from build123d import *

# Parameters (mm, degrees)
SKETCH3_R           = 7.5
SKETCH3_R_2         = 2.75
SKETCH3_W           = 30
SKETCH3_H           = 5.4
BOSS_EXTRUDE1_DEPTH = 5.4


with BuildPart() as part:
    # Sketch3 → Boss-Extrude1 (new body)
    with BuildSketch(Plane.XY):
        with BuildLine():
            Line((-242.5, 50), (207.5, 50))
            ThreePointArc((207.5, 50), (257.5, 0), (207.5, -50))
            Line((207.5, -50), (-242.5, -50))
            ThreePointArc((-242.5, -50), (-292.5, 0), (-242.5, 50))
        make_face()
        with Locations((-242.5, 0)):
            Circle(SKETCH3_R, mode=Mode.SUBTRACT)
        with Locations((207.5, 0)):
            Circle(SKETCH3_R, mode=Mode.SUBTRACT)
        with Locations((-226.332108181, 6.696960066)):
            Circle(SKETCH3_R_2, mode=Mode.SUBTRACT)
        with Locations((-226.332108181, -6.696960066)):
            Circle(SKETCH3_R_2, mode=Mode.SUBTRACT)
        with Locations((-235.803039934, -16.167891819)):
            Circle(SKETCH3_R_2, mode=Mode.SUBTRACT)
        with Locations((-249.196960066, -16.167891819)):
            Circle(SKETCH3_R_2, mode=Mode.SUBTRACT)
        with Locations((-258.667891819, -6.696960066)):
            Circle(SKETCH3_R_2, mode=Mode.SUBTRACT)
        with Locations((-258.667891819, 6.696960066)):
            Circle(SKETCH3_R_2, mode=Mode.SUBTRACT)
        with Locations((-249.196960066, 16.167891819)):
            Circle(SKETCH3_R_2, mode=Mode.SUBTRACT)
        with Locations((-235.803039934, 16.167891819)):
            Circle(SKETCH3_R_2, mode=Mode.SUBTRACT)
        with Locations((-134.5, -24)):
            Circle(SKETCH3_R_2, mode=Mode.SUBTRACT)
        with Locations((-154.5, -24)):
            Circle(SKETCH3_R_2, mode=Mode.SUBTRACT)
        with Locations((-168.5, -10)):
            Circle(SKETCH3_R_2, mode=Mode.SUBTRACT)
        with Locations((-168.5, 10)):
            Circle(SKETCH3_R_2, mode=Mode.SUBTRACT)
        with Locations((-154.5, 24)):
            Circle(SKETCH3_R_2, mode=Mode.SUBTRACT)
        with Locations((-134.5, 24)):
            Circle(SKETCH3_R_2, mode=Mode.SUBTRACT)
        with Locations((199.5, -24)):
            Circle(SKETCH3_R_2, mode=Mode.SUBTRACT)
        with Locations((219.5, -24)):
            Circle(SKETCH3_R_2, mode=Mode.SUBTRACT)
        with Locations((233.5, -10)):
            Circle(SKETCH3_R_2, mode=Mode.SUBTRACT)
        with Locations((233.5, 10)):
            Circle(SKETCH3_R_2, mode=Mode.SUBTRACT)
        with Locations((219.5, 24)):
            Circle(SKETCH3_R_2, mode=Mode.SUBTRACT)
        with Locations((199.5, 24)):
            Circle(SKETCH3_R_2, mode=Mode.SUBTRACT)
        with BuildLine():
            Line((115, 15), (150, 15))
            ThreePointArc((150, 15), (165, 0), (150, -15))
            Line((150, -15), (115, -15))
            ThreePointArc((115, -15), (100, 0), (115, 15))
        make_face(mode=Mode.SUBTRACT)
        with Locations((-227.5, 42.3)):
            Rectangle(SKETCH3_W, SKETCH3_H, mode=Mode.SUBTRACT)
        with Locations((-167.5, 42.3)):
            Rectangle(SKETCH3_W, SKETCH3_H, mode=Mode.SUBTRACT)
        with BuildLine():
            Line((14.924, 15), (49.924, 15))
            ThreePointArc((49.924, 15), (64.924, 0), (49.924, -15))
            Line((49.924, -15), (14.924, -15))
            ThreePointArc((14.924, -15), (-0.076, 0), (14.924, 15))
        make_face(mode=Mode.SUBTRACT)
        with BuildLine():
            Line((-85.152, 15), (-50.152, 15))
            ThreePointArc((-50.152, 15), (-35.152, 0), (-50.152, -15))
            Line((-50.152, -15), (-85.152, -15))
            ThreePointArc((-85.152, -15), (-100.152, 0), (-85.152, 15))
        make_face(mode=Mode.SUBTRACT)
        with Locations((-107.5, 42.3)):
            Rectangle(SKETCH3_W, SKETCH3_H, mode=Mode.SUBTRACT)
        with Locations((-47.5, 42.3)):
            Rectangle(SKETCH3_W, SKETCH3_H, mode=Mode.SUBTRACT)
        with Locations((12.5, 42.3)):
            Rectangle(SKETCH3_W, SKETCH3_H, mode=Mode.SUBTRACT)
        with Locations((72.5, 42.3)):
            Rectangle(SKETCH3_W, SKETCH3_H, mode=Mode.SUBTRACT)
        with Locations((132.5, 42.3)):
            Rectangle(SKETCH3_W, SKETCH3_H, mode=Mode.SUBTRACT)
        with Locations((192.5, 42.3)):
            Rectangle(SKETCH3_W, SKETCH3_H, mode=Mode.SUBTRACT)
        with Locations((192.5, -42.3)):
            Rectangle(SKETCH3_W, SKETCH3_H, mode=Mode.SUBTRACT)
        with Locations((132.5, -42.3)):
            Rectangle(SKETCH3_W, SKETCH3_H, mode=Mode.SUBTRACT)
        with Locations((72.5, -42.3)):
            Rectangle(SKETCH3_W, SKETCH3_H, mode=Mode.SUBTRACT)
        with Locations((12.5, -42.3)):
            Rectangle(SKETCH3_W, SKETCH3_H, mode=Mode.SUBTRACT)
        with Locations((-47.5, -42.3)):
            Rectangle(SKETCH3_W, SKETCH3_H, mode=Mode.SUBTRACT)
        with Locations((-107.5, -42.3)):
            Rectangle(SKETCH3_W, SKETCH3_H, mode=Mode.SUBTRACT)
        with Locations((-167.5, -42.3)):
            Rectangle(SKETCH3_W, SKETCH3_H, mode=Mode.SUBTRACT)
        with Locations((-227.5, -42.3)):
            Rectangle(SKETCH3_W, SKETCH3_H, mode=Mode.SUBTRACT)
    extrude(amount=BOSS_EXTRUDE1_DEPTH)


solid = part.part
The listing builds one solid part. Answer for the finished solid, in the listing's coordinates (mm). A direction names the side the tool comes from. Round coordinates to 2 decimals unless told otherwise and drop trailing zeros. Write each question's results on one line, items separated by ' | '. Start each with the question number.
1) Each of these flat-tipped pins is pushed along its axis until it touches: pin 1 (1.6 mm diameter, centred on y = 41.5, z = 2, fed in from +X); pin 2 (2.5 mm diameter, centred on y = -43.5, z = 3, fed in from -X); pin 3 (4 mm diameter, centred on x = -222.5, y = 31.5, fed in from -Z); pin 4 (2.5 mm diameter, centred on y = -42.5, z = 3.5, fed in from +X). Where does it stop, or does it pass through?
2) Straight lines are drawn through the part: probe 1 along Y at (x, z) = (-112, 3.2); probe 2 along X at (y, z) = (2.5, 1.5); probe 3 along Y at (x, z) = (-154.5, 3.5). For each, find the intervals that lie inside material, in ascending order.
3) Determine the mould class of faces 1 (the cylindrical face through (-292.488, -1.099, 2.662)), 2 (the cylindrical face through (-35.156, 0.33, 2.662)), 3 (the flat face through (-14, 1, 5.4)) for opening direction Y: pulls with the +Y half, pulls with the -Y half, needs draft (parallel to the pull), parting line crosses it, or undercut.
4) Find section A-A on z = 2.7. Count the separate pieces of the cut face and the enclosed holes in it, plus the area to 3 significant figures.
5) Which of the six approach directions +Z, -Z, +X, -X, +Y, -Y give full straight-line access (tool end or side, diameter ignored) to faces 4 (the flat face through (-14, 1, 0)), 5 (the cylindrical face through (-100.15, -0.33, 2.66))?
Final values:
1) pin 1: x = 236.54 | pin 2: x = -269.24 | pin 3: z = 0 | pin 4: x = 235.76
2) probe 1: -50 to -45, -39.6 to 39.6, 45 to 50 | probe 2: -292.44 to -249.57, -235.43 to -99.94, -35.36 to 0.13, 64.71 to 100.21, 164.79 to 200.43, 214.57 to 257.44 | probe 3: -50 to -45, -39.6 to -26.75, -21.25 to 21.25, 26.75 to 39.6, 45 to 50
3) face 1: parting line crosses it | face 2: undercut | face 3: needs draft
4) separate pieces: 1 | enclosed holes: 41 | area: 44,200 mm²
5) face 4: -Z, +X, -X, +Y, -Y | face 5: +Z, -Z
